Work out the finished part from the listing and answer in its coordinate system (mm). Coordinates: 2 decimals unless noted, no trailing zeros. Write each loop counter-clockwise with the first axis right and the second up, starting at its lowest first coordinate (ties: lowest second). Pieces come first, ordered by that corner, then holes. Notation, with made-up numbers: (-30, 20) - (27, 20) arc R26 ccw to (27, 47) - close; hole circle Ø4 at (7, 54.5). An arc over 180 degrees is marked (long way). Use a Markdown table: item, result. Add a question column.
(1) Find the intervals of material crossed by line 1 (Z direction, x = 32, y = 90); line 2 (Z direction, x = -40, y = 73.5), in increasing order. Write a range as from..to.
(2) The part is cut by section B-B, the plane z = 41.5. Give the vertices of the cut face in (x, y), then the cut area to 3 significant figures.
(3) Given pin 1 Ø1.5 at (y, z) = (-51.5, 39) entering from +X, flat-ended and moving along its own axis, determine where the tip first touches the part or whether it passes through.
(4) The part is cut by section A-A, the plane y = 19. Give the vertices of the cut face in (x, z).
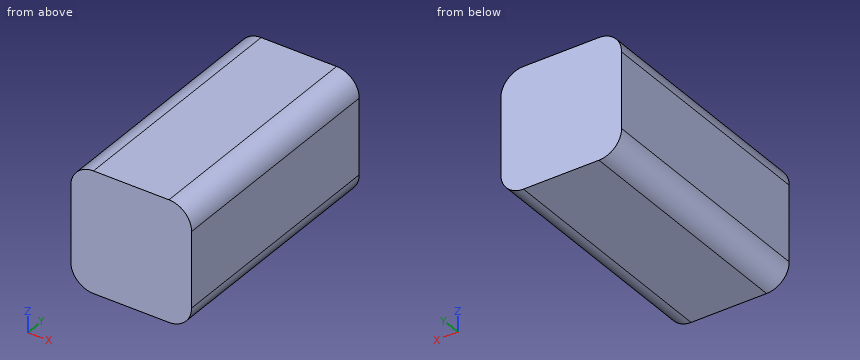
from build123d import *

# Parameters (mm, degrees)
F0_W          = 101.6
F0_H          = 101.6
F1_DEPTH      = 101.6
F1_DEPTH_BACK = 101.6
F2_R          = 19.05
F3_R          = 2.738729
F4_DEPTH      = 19.304


with BuildPart() as f1:
    # F0 (on Front) → F1 (new body, two sides)
    with BuildSketch(Plane.XZ) as f1_sk:
        Rectangle(F0_W, F0_H)
    extrude(amount=F1_DEPTH)
    extrude(f1_sk.sketch, amount=-F1_DEPTH_BACK)

    # F2
    f2_edges = [f1.edges().sort_by_distance(p)[0] for p in [
        (-50.8, 0, 50.8),
        (50.8, 0, 50.8),
        (50.8, 0, -50.8),
        (-50.8, 0, -50.8),
    ]]
    fillet(f2_edges, radius=F2_R)

    # F3 (on face) → F4 (join)
    with BuildSketch(Plane(origin=(0, 0, -50.8), x_dir=(1, 0, 0), z_dir=(0, 0, -1))):
        with Locations((-22.506165, 95.329402)):
            Circle(F3_R)
    extrude(amount=-F4_DEPTH)


solid = f1.part
Model answer:
| question | item | result |
|---|---|---|
| 1 | line 1 | -50.8..50.8 |
| 1 | line 2 | -48.92..48.92 |
| 2 | outline | (-48.12, -101.6) - (48.12, -101.6) - (48.12, 101.6) - (-48.12, 101.6) - close |
| 2 | area | 19,600 mm^2 |
| 3 | pin 1 | x = 49.66 |
| 4 | outline | (-50.8, -31.75) arc R19.05 ccw to (-31.75, -50.8) - (31.75, -50.8) arc R19.05 ccw to (50.8, -31.75) - (50.8, 31.75) arc R19.05 ccw to (31.75, 50.8) - (-31.75, 50.8) arc R19.05 ccw to (-50.8, 31.75) - close |
